Could you check a few things on this drawing? It's one solid part, dimensions in mm from its lowest x, y, z. Round coordinates to 2 decimals unless told otherwise and drop trailing zeros. Loops run counter-clockwise (first coordinate to the right, second up) from the corner with the lowest first, then second, coordinate; pieces in that order, holes last. Notation, with made-up numbers: M 20,52.25 L 47,52.25 A11 cw 47,58.25 Z; hole C 44,-11 d3. An arc over 180 degrees is marked long. Return JSON: item names as keys, results as strings.
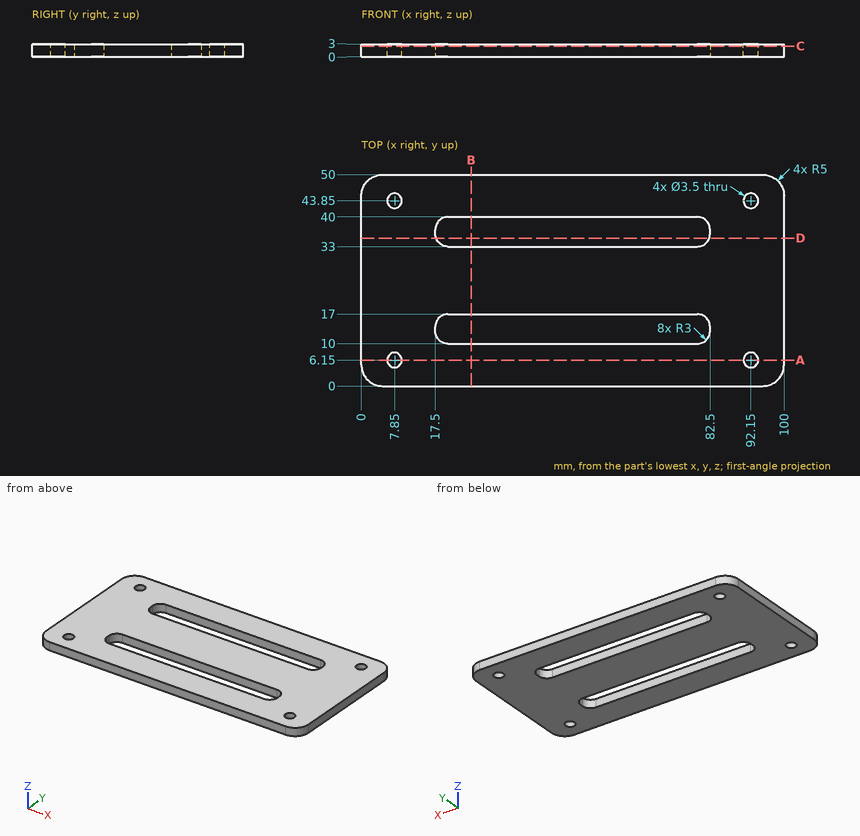
Q1. Suppose I cut it at B-B, the plane x = 26. Please give me the cut outline in (y, z), plus the area to 3 significant figures.
Results:
{"outline": "M 0,0 L 10,0 L 10,3 L 0,3 Z; M 17,0 L 33,0 L 33,3 L 17,3 Z; M 40,0 L 50,0 L 50,3 L 40,3 Z", "area": "108 mm2"}
Q2. Suppose I cut it at A-A, the plane y = 6.15. Please give me the cut outline in (x, z).
Results:
{"outline": "M 0,0 L 6.1,0 L 6.1,3 L 0,3 Z; M 9.6,0 L 90.4,0 L 90.4,3 L 9.6,3 Z; M 93.9,0 L 100,0 L 100,3 L 93.9,3 Z"}
Q3. If I drill on line 1 along X through (y, z) = (6, 2.4); line 2 along Y through (x, z) = (92.15, 1.3); line 3 along Y through (x, z) = (76, 2.55), over which ranges is the centre line in solid material (lowest first)?
Results:
{"line 1": "x = 0 to 6.11, 9.59 to 90.41, 93.89 to 100", "line 2": "y = 0 to 4.4, 7.9 to 42.1, 45.6 to 50", "line 3": "y = 0 to 10, 17 to 33, 40 to 50"}
Q4. Suppose I cut it at C-C, the plane z = 2.5. Please give me the cut outline in (x, y), plus the area to 3 significant figures.
Results:
{"outline": "M 0,5 A5 ccw 5,0 L 95,0 A5 ccw 100,5 L 100,45 A5 ccw 95,50 L 5,50 A5 ccw 0,45 Z; hole C 7.85,6.15 d3.5; hole C 7.85,43.85 d3.5; hole M 17.5,13 A3 ccw 20.5,10 L 79.5,10 A3 ccw 82.5,13 L 82.5,14 A3 ccw 79.5,17 L 20.5,17 A3 ccw 17.5,14 Z; hole M 17.5,36 A3 ccw 20.5,33 L 79.5,33 A3 ccw 82.5,36 L 82.5,37 A3 ccw 79.5,40 L 20.5,40 A3 ccw 17.5,37 Z; hole C 92.15,6.15 d3.5; hole C 92.15,43.85 d3.5", "area": "4,050 mm2"}
Q5. Suppose I cut it at D-D, the plane y = 35. Please give me the cut outline in (x, z).
Results:
{"outline": "M 0,0 L 17.67,0 L 17.67,3 L 0,3 Z; M 82.33,0 L 100,0 L 100,3 L 82.33,3 Z"}
